Could you check a few things on this model? Use its own coordinates, in mm. Give positions to 0.01 mm unless a question says otherwise; leave off trailing zeros. Order: outer loops, then holes, each group sorted by start corner. A loop starts at its lowest first (then second) coordinate and runs counter-clockwise, first axis right, second up. Notation, with made-up numbers: (4.25, -16) -> (46.25, -16) arc R17 ccw to (46.25, -3) -> close; hole circle Ø9 at (49.25, 45). An arc over 180 degrees is marked (long way). Write each question's results on one line, items separated by ' | '.
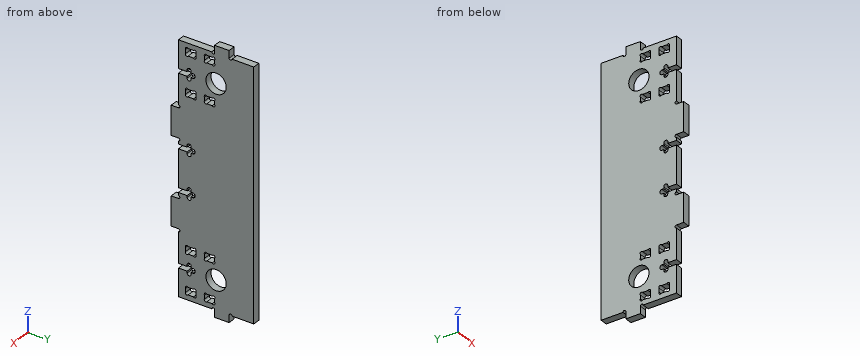
```python
from build123d import *

# Parameters (mm, degrees)
SKETCH_1_W          = 170
SKETCH_1_H          = 52
EXTRUDE_1_DEPTH     = 5
SKETCH_2_R          = 7
CUT_EXTRUDE_1_DEPTH = 10
SKETCH_3_W          = 20
SKETCH_3_H          = 5
EXTRUDE_2_DEPTH     = 5
CUT_EXTRUDE_2_DEPTH = 10
SKETCH_8_W          = 5
SKETCH_8_H          = 10
EXTRUDE_3_DEPTH     = 5
SKETCH_7_R          = 1
CUT_EXTRUDE_3_DEPTH = 10
SKETCH_10_W         = 5
SKETCH_10_H         = 7
CUT_EXTRUDE_4_DEPTH = 10
SKETCH_11_R         = 1
CUT_EXTRUDE_5_DEPTH = 10


with BuildPart() as part:
    # 스케치1 → 보스-돌출1 (new body)
    with BuildSketch(Plane(origin=(0, 0, 0), x_dir=(0, 0, -1), z_dir=(1, 0, 0))):
        with Locations((85, 26)):
            Rectangle(SKETCH_1_W, SKETCH_1_H)
    extrude(amount=EXTRUDE_1_DEPTH)

    # 스케치2 → 컷-돌출1 (cut)
    with BuildSketch(Plane(origin=(5, 0, 0), x_dir=(0, 0, -1), z_dir=(1, 0, 0))):
        with Locations((150, 26)):
            Circle(SKETCH_2_R)
        with Locations((20, 26)):
            Circle(SKETCH_2_R)
    extrude(amount=-CUT_EXTRUDE_1_DEPTH, mode=Mode.SUBTRACT)

    # 스케치3 → 보스-돌출2 (add)
    with BuildSketch(Plane(origin=(5, 0, 0), x_dir=(0, 0, -1), z_dir=(1, 0, 0))):
        with Locations((55, -2.5)):
            Rectangle(SKETCH_3_W, SKETCH_3_H)
        with Locations((115, -2.5)):
            Rectangle(SKETCH_3_W, SKETCH_3_H)
    extrude(amount=-EXTRUDE_2_DEPTH)

    # 스케치6 → 컷-돌출2 (cut)
    with BuildSketch(Plane(origin=(5, 0, 0), x_dir=(0, 0, -1), z_dir=(1, 0, 0))):
        with BuildLine():
            Line((151, 0), (151, 6))
            Line((151, 6), (152.2, 6))
            ThreePointArc((152.2, 6), (153.6, 7.4), (152.2, 8.8))
            Line((152.2, 8.8), (151, 8.8))
            Line((151, 8.8), (151, 10))
            ThreePointArc((151, 10), (149.45, 11.55), (147.9, 10))
            Line((147.9, 10), (147.9, 8.8))
            Line((147.9, 8.8), (146.7, 8.8))
            ThreePointArc((146.7, 8.8), (145.3, 7.4), (146.7, 6))
            Line((146.7, 6), (147.9, 6))
            Line((147.9, 6), (147.9, 0))
            Line((147.9, 0), (151, 0))
        make_face()
        with BuildLine():
            Line((101, 0), (101, 6))
            Line((101, 6), (102.2, 6))
            ThreePointArc((102.2, 6), (103.6, 7.4), (102.2, 8.8))
            Line((102.2, 8.8), (101, 8.8))
            Line((101, 8.8), (101, 10))
            ThreePointArc((101, 10), (99.45, 11.55), (97.9, 10))
            Line((97.9, 10), (97.9, 8.8))
            Line((97.9, 8.8), (96.7, 8.8))
            ThreePointArc((96.7, 8.8), (95.3, 7.4), (96.7, 6))
            Line((96.7, 6), (97.9, 6))
            Line((97.9, 6), (97.9, 0))
            Line((97.9, 0), (101, 0))
        make_face()
        with BuildLine():
            Line((67.8, 6), (69, 6))
            Line((69, 6), (69, 0))
            Line((69, 0), (72.1, 0))
            Line((72.1, 0), (72.1, 6))
            Line((72.1, 6), (73.3, 6))
            ThreePointArc((73.3, 6), (74.7, 7.4), (73.3, 8.8))
            Line((73.3, 8.8), (72.1, 8.8))
            Line((72.1, 8.8), (72.1, 10))
            ThreePointArc((72.1, 10), (70.55, 11.55), (69, 10))
            Line((69, 10), (69, 8.8))
            Line((69, 8.8), (67.8, 8.8))
            ThreePointArc((67.8, 8.8), (66.4, 7.4), (67.8, 6))
        make_face()
        with BuildLine():
            Line((17.8, 6), (19, 6))
            Line((19, 6), (19, 0))
            Line((19, 0), (22.1, 0))
            Line((22.1, 0), (22.1, 6))
            Line((22.1, 6), (23.3, 6))
            ThreePointArc((23.3, 6), (24.7, 7.4), (23.3, 8.8))
            Line((23.3, 8.8), (22.1, 8.8))
            Line((22.1, 8.8), (22.1, 10))
            ThreePointArc((22.1, 10), (20.55, 11.55), (19, 10))
            Line((19, 10), (19, 8.8))
            Line((19, 8.8), (17.8, 8.8))
            ThreePointArc((17.8, 8.8), (16.4, 7.4), (17.8, 6))
        make_face()
    extrude(amount=-CUT_EXTRUDE_2_DEPTH, mode=Mode.SUBTRACT)

    # 스케치8 → 보스-돌출3 (add)
    with BuildSketch(Plane(origin=(5, 0, 0), x_dir=(0, 0, -1), z_dir=(1, 0, 0))):
        with Locations((172.5, 30)):
            Rectangle(SKETCH_8_W, SKETCH_8_H)
        with Locations((-2.5, 30)):
            Rectangle(SKETCH_8_W, SKETCH_8_H)
    extrude(amount=-EXTRUDE_3_DEPTH)

    # 스케치7 → 컷-돌출3 (cut)
    with BuildSketch(Plane(origin=(5, 0, 0), x_dir=(0, 0, -1), z_dir=(1, 0, 0))):
        with Locations((66, 0)):
            Circle(SKETCH_7_R)
        with Locations((44, 0)):
            Circle(SKETCH_7_R)
        with Locations((104, 0)):
            Circle(SKETCH_7_R)
        with Locations((126, 0)):
            Circle(SKETCH_7_R)
        with Locations((170, 36)):
            Circle(SKETCH_7_R)
        with Locations((170, 24)):
            Circle(SKETCH_7_R)
        with Locations((0, 36)):
            Circle(SKETCH_7_R)
        with Locations((0, 24)):
            Circle(SKETCH_7_R)
    extrude(amount=-CUT_EXTRUDE_3_DEPTH, mode=Mode.SUBTRACT)

    # 스케치10 → 컷-돌출4 (cut)
    with BuildSketch(Plane.ZY):
        with Locations((-164, 21.5)):
            Rectangle(SKETCH_10_W, SKETCH_10_H)
        with Locations((-137, 21.5)):
            Rectangle(SKETCH_10_W, SKETCH_10_H)
        with Locations((-164, 8.5)):
            Rectangle(SKETCH_10_W, SKETCH_10_H)
        with Locations((-137, 8.5)):
            Rectangle(SKETCH_10_W, SKETCH_10_H)
        with Locations((-33, 8.5)):
            Rectangle(SKETCH_10_W, SKETCH_10_H)
        with Locations((-6, 8.5)):
            Rectangle(SKETCH_10_W, SKETCH_10_H)
        with Locations((-33, 21.5)):
            Rectangle(SKETCH_10_W, SKETCH_10_H)
        with Locations((-6, 21.5)):
            Rectangle(SKETCH_10_W, SKETCH_10_H)
    extrude(amount=-CUT_EXTRUDE_4_DEPTH, mode=Mode.SUBTRACT)

    # 스케치11 → 컷-돌출5 (cut)
    with BuildSketch(Plane(origin=(5, 0, 0), x_dir=(0, 0, -1), z_dir=(1, 0, 0))):
        with Locations((165.918761806, 24.186266529)):
            Circle(SKETCH_11_R)
        with Locations((162.081238194, 24.186266529)):
            Circle(SKETCH_11_R)
        with Locations((165.918761806, 18.813733471)):
            Circle(SKETCH_11_R)
        with Locations((162.081238194, 18.813733471)):
            Circle(SKETCH_11_R)
        with Locations((138.918761806, 18.813733471)):
            Circle(SKETCH_11_R)
        with Locations((135.081238194, 18.813733471)):
            Circle(SKETCH_11_R)
        with Locations((138.918761806, 24.186266529)):
            Circle(SKETCH_11_R)
        with Locations((135.081238194, 24.186266529)):
            Circle(SKETCH_11_R)
        with Locations((135.081238194, 5.813733471)):
            Circle(SKETCH_11_R)
        with Locations((138.918761806, 5.813733471)):
            Circle(SKETCH_11_R)
        with Locations((135.081238194, 11.186266529)):
            Circle(SKETCH_11_R)
        with Locations((138.918761806, 11.186266529)):
            Circle(SKETCH_11_R)
        with Locations((162.081238194, 11.186266529)):
            Circle(SKETCH_11_R)
        with Locations((165.918761806, 11.186266529)):
            Circle(SKETCH_11_R)
        with Locations((162.081238194, 5.813733471)):
            Circle(SKETCH_11_R)
        with Locations((165.918761806, 5.813733471)):
            Circle(SKETCH_11_R)
        with Locations((4.081238194, 5.813733471)):
            Circle(SKETCH_11_R)
        with Locations((7.918761806, 5.813733471)):
            Circle(SKETCH_11_R)
        with Locations((4.081238194, 11.186266529)):
            Circle(SKETCH_11_R)
        with Locations((7.918761806, 11.186266529)):
            Circle(SKETCH_11_R)
        with Locations((31.081238194, 11.186266529)):
            Circle(SKETCH_11_R)
        with Locations((34.918761806, 11.186266529)):
            Circle(SKETCH_11_R)
        with Locations((31.081238194, 5.813733471)):
            Circle(SKETCH_11_R)
        with Locations((34.918761806, 5.813733471)):
            Circle(SKETCH_11_R)
        with Locations((34.918761806, 24.186266529)):
            Circle(SKETCH_11_R)
        with Locations((31.081238194, 24.186266529)):
            Circle(SKETCH_11_R)
        with Locations((34.918761806, 18.813733471)):
            Circle(SKETCH_11_R)
        with Locations((31.081238194, 18.813733471)):
            Circle(SKETCH_11_R)
        with Locations((7.918761806, 18.813733471)):
            Circle(SKETCH_11_R)
        with Locations((4.081238194, 18.813733471)):
            Circle(SKETCH_11_R)
        with Locations((7.918761806, 24.186266529)):
            Circle(SKETCH_11_R)
        with Locations((4.081238194, 24.186266529)):
            Circle(SKETCH_11_R)
    extrude(amount=-CUT_EXTRUDE_5_DEPTH, mode=Mode.SUBTRACT)


solid = part.part
```
Q1. Suppose I cut it at B-B on y = 29. Please give me the cut outline in (x, z), and give its area (3 significant figures).
Here are the results:
outline: (0, -175) -> (5, -175) -> (5, -156.32) -> (0, -156.32) -> close; (0, -143.68) -> (5, -143.68) -> (5, -26.32) -> (0, -26.32) -> close; (0, -13.68) -> (5, -13.68) -> (5, 5) -> (0, 5) -> close | area: 774 mm²
Q2. Suppose I cut it at A-A on z = -20.55. Please give me the cut outline in (x, y), and give its area (3 significant figures).
Here are the results:
outline: (0, 11.55) -> (5, 11.55) -> (5, 19.02) -> (0, 19.02) -> close; (0, 32.98) -> (5, 32.98) -> (5, 52) -> (0, 52) -> close | area: 132 mm²
Q3. I'm going to push flat-ended pins straight in: pin 1 Ø1 at (x, y) = (3.5, 9.5) entering from +Z; pin 2 Ø1.5 at (x, z) = (3.5, -11) entering from -Y; pin 3 Ø1.5 at (x, y) = (3, -1.5) entering from +Z. Where does each tip first touch, or does it pass through?
Here are the results:
pin 1: stops at z = 0 | pin 2: stops at y = 0 | pin 3: stops at z = -45
Q4. Suppose I cut it at C-C on x = 4. State how many separate pieces and enclosed holes the cut face has, and give its area (3 significant figures).
Here are the results:
separate pieces: 1 | enclosed holes: 10 | area: 8,330 mm²
Q5. Suppose I cut it at D-D on y = 41. Please give me the cut outline in (x, z), and give its area (3 significant figures).
Here are the results:
outline: (0, -170) -> (5, -170) -> (5, 0) -> (0, 0) -> close | area: 850 mm²
Q6. I need wall thicknesses on line 1 along Z through (x, y) = (1.55, 26.5); line 2 along Y through (x, z) = (0.4, -67.5); line 3 along Z through (x, y) = (3.9, -0.5). Which ranges of each line are inside material? Lowest first, please.
Here are the results:
line 1: z = -175 to -156.98, -143.02 to -26.98, -13.02 to 5 | line 2: y = 0 to 6.03, 8.77 to 52 | line 3: z = -125 to -105, -65 to -45
